Source: CAD feature listing. Evaluate the final solid. Frame: model axes, mm. A direction names the side the tool comes from. Give positions to 0.01 mm unless a question says otherwise; leave off trailing zeros. Order: outer loops, then holes, each group sorted by start corner. A loop starts at its lowest first (then second) coordinate and runs counter-clockwise, first axis right, second up.
from build123d import *

# Parameters (mm, degrees)
AUFSATZ_LINEAR_AUSTRAGEN1_DEPTH = 35
SKIZZE3_R                       = 6
AUFSATZ_LINEAR_AUSTRAGEN2_DEPTH = 5
SKIZZE4_R                       = 6.5
AUFSATZ_LINEAR_AUSTRAGEN3_DEPTH = 0.1
SKIZZE9_R                       = 1.425
SCHNITT_LINEAR_AUSTRAGEN2_DEPTH = 10
SKIZZE10_R                      = 2.25
AUFSATZ_LINEAR_AUSTRAGEN4_DEPTH = 7
VERRUNDUNG1_R                   = 5
VERRUNDUNG2_R                   = 1


with BuildPart() as part:
    # Skizze1 → Aufsatz-Linear austragen1 (new body)
    with BuildSketch(Plane(origin=(0, 0, 0), x_dir=(0, 0, -1), z_dir=(1, 0, 0))):
        Polygon((0, 0), (22.497566339, 0), (26.82, 0), (26.82, 66.811555509), (22.497566339, 66.811555509), (0, 40), align=None)
    extrude(amount=AUFSATZ_LINEAR_AUSTRAGEN1_DEPTH)

    # Skizze3 → Aufsatz-Linear austragen2 (add)
    with BuildSketch(Plane(origin=(0, 16.527036447, 19.69615506), x_dir=(1, 0, 0), z_dir=(0, 0.6427876096865378, 0.7660444431189795))):
        with Locations(Location((17.5, 48.141777725, 0), (0, 0, 90))):
            Circle(SKIZZE3_R)
    extrude(amount=AUFSATZ_LINEAR_AUSTRAGEN2_DEPTH)

    # Skizze4 → Aufsatz-Linear austragen3 (add)
    with BuildSketch(Plane(origin=(0, 16.527036447, 19.69615506), x_dir=(1, 0, 0), z_dir=(0, 0.6427876096865378, 0.7660444431189795))):
        with Locations(Location((17.5, 48.141777725, 0), (0, 0, 90))):
            Circle(SKIZZE4_R)
    extrude(amount=AUFSATZ_LINEAR_AUSTRAGEN3_DEPTH)

    # Skizze9 → Schnitt-Linear austragen2 (cut)
    with BuildSketch(Plane.XZ):
        with Locations(Location((17.498844944, -21.644236877, 0), (0, 0, 270))):
            Circle(SKIZZE9_R)
    extrude(amount=-SCHNITT_LINEAR_AUSTRAGEN2_DEPTH, mode=Mode.SUBTRACT)

    # Skizze10 → Aufsatz-Linear austragen4 (add)
    # profile 1 of 2: a face of its own
    with BuildSketch(Plane.XZ):
        Polygon((35, -26.82), (36.222689888, -26.82), (36.222689888, -23.396698607), (46.898151193, 14.806878364), (27.636053566, 20.189405189), (21.994403466, 0), align=None)
        with Locations(Location((35.132608407, 9.859567437, 0), (0, 0, 270))):
            Circle(SKIZZE10_R, mode=Mode.SUBTRACT)
    # profile 2 of 2: a face of its own
    with BuildSketch(Plane.XZ):
        Polygon((-1.222689888, -26.82), (-1.222689888, -23.396698607), (-11.898151193, 14.806878364), (7.363946434, 20.189405189), (13.005596534, 0), (0, -26.82), align=None)
        with Locations(Location((-0.132608407, 9.859567437, 0), (0, 0, 90))):
            Circle(SKIZZE10_R, mode=Mode.SUBTRACT)
    extrude(amount=-AUFSATZ_LINEAR_AUSTRAGEN4_DEPTH)

    # Verrundung1
    verrundung1_edges = [part.edges().sort_by_distance(p)[0] for p in [
        (6.502798267, 7, 0),
        (28.497201733, 7, 0),
        (35, 7, -13.41),
        (0, 7, -13.41),
        (-11.898151193, 3.5, 14.806878364),
        (7.363946434, 3.5, 20.189405189),
        (46.898151193, 3.5, 14.806878364),
        (27.636053566, 3.5, 20.189405189),
        (21.994403466, 3.5, 0),
        (13.005596534, 3.5, 0),
    ]]
    fillet(verrundung1_edges, radius=VERRUNDUNG1_R)

    # Verrundung2
    verrundung2_edges = [part.edges().sort_by_distance(p)[0] for p in [
        (36.222689888, 4.362018901, -26.82),
        (-1.222689888, 4.362018901, -26.82),
    ]]
    fillet(verrundung2_edges, radius=VERRUNDUNG2_R)


solid = part.part
1) First-contact query: pin 1 Ø10.5 at (x, y) = (21.5, 13.5) entering from +Z; pin 2 Ø1.9 at (y, z) = (4.5, -24.5) entering from -X; pin 3 Ø11 at (x, z) = (30.5, 5) entering from +Y; pin 4 Ø3 at (x, z) = (32, -9.5) entering from -Y. Flat tips, straight axial feed; report the tip coordinate or a pass-through.
Checks:
pin 1: stops at z = 1.67
pin 2: stops at x = -1.22
pin 3: stops at y = 40.6
pin 4: stops at y = 0
2) Section query A-A on x = 21. Output: boundary loops of the cut face in (y, z), and give its area (3 significant figures).
Checks:
outline: (0, -26.82) - (66.81, -26.82) - (66.81, -22.5) - (57.6, -14.77) - (57.67, -14.69) - (57.2, -14.3) - (60.35, -10.55) - (52.89, -4.29) - (49.74, -8.04) - (49.27, -7.65) - (49.21, -7.73) - (40, 0) - (12, 0) arc R5 cw to (9.2, 0.86) - (0, 0.86) - close
area: 1,550 mm2
3) Section query C-C on z = -1. Output: boundary loops of the cut face in (x, y), and give its area (3 significant figures).
Checks:
outline: (-7.48, 0) - (42.48, 0) - (42.48, 7) - (40, 7) arc R5 cw to (35, 12) - (35, 41.19) - (0, 41.19) - (0, 12) arc R5 cw to (-5, 7) - (-7.48, 7) - close
area: 1,560 mm2
4) Reachability of faces 1 (the face through (10.324, 3.542, 9.596)), 2 (the face through (36.223, 4, -25)), 3 (the face through (17.56, 4.93, -20.22)) from +Z, -Z, +X, -X, +Y, -Y: full face, straight path, thin tool, end or side. Return the list, or none.
Checks:
face 1: +Z, +Y, -Y
face 2: -Z, +X, +Y, -Y
face 3: -Y
5) Section query B-B on y = 30. Output: boundary loops of the cut face in (x, z).
Checks:
outline: (0, -26.82) - (35, -26.82) - (35, 0) - (0, 0) - close
6) Pull-direction query (Z, two-part tool) for faces 4 (the face through (24.676, 3.542, 9.596)), 5 (the face through (33, 7, 11)), 6 (the face through (1.236, 3.451, 8.074)), 7 (the face through (11.55, 54.42, -8.82)); classes: +Z half, -Z half, draft (parallel to the pull), parting line (faces both ways), or undercut.
Checks:
face 4: +Z half
face 5: draft
face 6: undercut
face 7: undercut
7) Ray query, L1, parallel to X at y = 43, z = -6; L2, parallel to Y at x = 16, z = -6.5; L3, parallel to Z at x = 22, y = 39. Return the intervals inside material, ascending.
Checks:
L1: x = 0 to 35
L2: y = 0 to 47.75, 49.81 to 55.53
L3: z = -26.82 to 0
8) Section query D-D on x = 6. Output: boundary loops of the cut face in (y, z).
Checks:
outline: (0, -26.82) - (66.81, -26.82) - (66.81, -22.5) - (40, 0) - (12, 0) arc R5 cw to (7, 5) - (7, 18.56) - (0, 18.56) - close
